```python
from build123d import *

# Parameters (mm, degrees)
ESBO_O2_OUTSIDE_W          = 42.476
ESBO_O2_OUTSIDE_H          = 42.476
ESBO_O2_OUTSIDE_W_2        = 28
ESBO_O2_OUTSIDE_H_2        = 15
CORTE_EXTRUS_O1_DEPTH      = 25.1
CORTE_EXTRUS_O1_DEPTH_BACK = 25.1
CORTE_EXTRUS_O2_DEPTH      = 16


with BuildPart() as part:
    # Esboço1 → Revolução1 (revolve)
    with BuildSketch(Plane.XY):
        with BuildLine():
            Line((0, 24.1), (0, -24.1))
            ThreePointArc((0, -24.1), (9.899494937, -19.999494937), (14, -10.1))
            Line((14, -10.1), (9.9, -10.1))
            Line((9.9, -10.1), (9.9, 10.1))
            Line((9.9, 10.1), (14, 10.1))
            ThreePointArc((14, 10.1), (9.899494937, 19.999494937), (0, 24.1))
        make_face()
    revolve(axis=Axis((0, -24.1, 0), (0, 1, 0)))

    # Esboço2 outside → Corte-extrusão1 (cut, two sides)
    with BuildSketch(Plane(origin=(0, 0, 0), x_dir=(1, 0, 0), z_dir=(0, 1, 0))) as corte_extrus_o1_sk:
        Rectangle(ESBO_O2_OUTSIDE_W, ESBO_O2_OUTSIDE_H)
        Rectangle(ESBO_O2_OUTSIDE_W_2, ESBO_O2_OUTSIDE_H_2, mode=Mode.SUBTRACT)
    extrude(amount=CORTE_EXTRUS_O1_DEPTH, mode=Mode.SUBTRACT)
    extrude(corte_extrus_o1_sk.sketch, amount=-CORTE_EXTRUS_O1_DEPTH_BACK, mode=Mode.SUBTRACT)

    # Esboço3 → Corte-extrusão2 (cut, through all)
    with BuildSketch(Plane(origin=(0, 0, -7.5), x_dir=(-1, 0, 0), z_dir=(0, 0, -1))):
        with BuildLine():
            Line((5, 24.1), (5, 9.6))
            ThreePointArc((5, 9.6), (0, 4.6), (-5, 9.6))
            Line((-5, 9.6), (-5, 24.1))
            ThreePointArc((-5, 24.1), (0, 29.1), (5, 24.1))
        make_face()
        with BuildLine():
            Line((-5, -24.1), (-5, -9.6))
            ThreePointArc((-5, -9.6), (0, -4.6), (5, -9.6))
            Line((5, -9.6), (5, -24.1))
            ThreePointArc((5, -24.1), (0, -29.1), (-5, -24.1))
        make_face()
    extrude(amount=-CORTE_EXTRUS_O2_DEPTH, mode=Mode.SUBTRACT)


solid = part.part
```
Geometry check sheet. Reference: the model listing, model coordinates, mm. A direction names the side the tool comes from. Give positions to 0.01 mm unless a question says otherwise; leave off trailing zeros. Write each loop counter-clockwise with the first axis right and the second up, starting at its lowest first coordinate (ties: lowest second). Pieces come first, ordered by that corner, then holes.
1) Section check B-B, the plane z = 0.5. Record the boundary of the cut face in (x, y).
2) Section check A-A, the plane y = -14.5. Record the boundary of the cut face in (x, z), and give its area (3 significant figures).
3) Gauge pin test, flat ends, axial feed: pin 1 (8 mm diameter, centred on x = -10.5, z = -4.5, fed in from -Y); pin 2 (4 mm diameter, centred on y = -17, z = 3.5, fed in from -X); pin 3 (4 mm diameter, centred on y = 8.5, z = 2, fed in from -X); pin 4 (5 mm diameter, centred on x = 4.5, y = -11, fed in from -Z). Record the tip position at first contact, or that the pin passes through.
4) Release check for a two-part mould opening along X. For faces 6 (the flat face through (-5, -16, 0)), 7 (the flat face through (-11, -10.1, 0)), 8 (the cylindrical face through (9.9, 0.1, 0.1)) record: pulls with the +X half, pulls with the -X half, needs draft (parallel to the pull), parting line crosses it, or undercut.
5) Section check C-C, the plane x = 0. Record the boundary of the cut face in (y, z).
6) Access from +Z, -Z, +X, -X, +Y, -Y to the whole of each face (thin tool, end or side, straight path). Record for faces 1 (the flat face through (11, 10.1, 0)), 2 (the flat face through (-5, 16, 0)), 3 (the cylindrical face through (-9.9, 0.1, -0.1)), 4 (the flat face through (5, -16, 0)), 5 (the flat face through (0, 0, 7.5)).
7) Material ranges on L1, parallel to X at y = 8, z = -1.5; L2, parallel to Y at x = 10.25, z = -2.25; L3, parallel to X at y = -17, z = 6.5, recorded low to high.
8) Section check D-D, the plane y = -9. Record the boundary of the cut face in (x, z).
Computed:
1. outline: (-13.99, -10.1) arc R13.99 ccw to (-5, -23.17) - (-5, -9.6) arc R5 cw to (5, -9.6) - (5, -23.17) arc R13.99 ccw to (13.99, -10.1) - (9.89, -10.1) - (9.89, 10.1) - (13.99, 10.1) arc R13.99 ccw to (5, 23.17) - (5, 9.6) arc R5 cw to (-5, 9.6) - (-5, 23.17) arc R13.99 ccw to (-13.99, 10.1) - (-9.89, 10.1) - (-9.89, -10.1) - close
2. outline: (-10.97, -7.5) - (-5, -7.5) - (-5, 7.5) - (-10.97, 7.5) arc R13.29 ccw to start; (5, -7.5) - (10.97, -7.5) arc R13.29 ccw to (10.97, 7.5) - (5, 7.5) - close
2. area: 226 mm2
3. pin 1: stops at y = -21.97
3. pin 2: stops at x = -12.77
3. pin 3: stops at x = -13.98
3. pin 4: stops at z = -7.5
4. face 6: undercut
4. face 7: needs draft
4. face 8: pulls with the +X half
5. outline: (-4.6, -7.5) - (4.6, -7.5) - (4.6, 7.5) - (-4.6, 7.5) - close
6. face 1: +X
6. face 2: +Z, -Z, +Y
6. face 3: -X
6. face 4: +Z, -Z, -Y
6. face 5: +Z, +X, -X, +Y, -Y
7. L1: x = -9.79 to -4.74, 4.74 to 9.79
7. L2: y = -19.37 to -10.1, 10.1 to 19.37
7. L3: x = -10.3 to -5, 5 to 10.3
8. outline: (-6.46, -7.5) - (-4.96, -7.5) - (-4.96, 7.5) - (-6.46, 7.5) arc R9.9 ccw to start; (4.96, -7.5) - (6.46, -7.5) arc R9.9 ccw to (6.46, 7.5) - (4.96, 7.5) - close
